Geometry: see drawing. Coordinates: mm, zero at the bounding-box minimum. Round coordinates to 2 decimals unless told otherwise and drop trailing zeros. Loops run counter-clockwise (first coordinate to the right, second up) from the corner with the lowest first, then second, coordinate; pieces in that order, holes last.
(1) Material intervals for probe 1 along X at (y, z) = (19, 93) (1 decimal); probe 2 along Z at (x, y) = (61, 16.5) (1 decimal); probe 3 along Z at (x, y) = (69, 3.5) (1 decimal), sorted ascending.
(2) Section B-B, the plane x = 38.5. Return the cut outline in (y, z), plus the area to 3 significant figures.
(3) Mould query, pull axis Z, two halves, no side actions, for the marked faces 1, 2 and 3. Classes: pulls with the +Z half, pulls with the -Z half, needs draft (parallel to the pull), parting line crosses it, or undercut.
(4) First-contact query: pin 1 Ø3 at (x, y) = (69.5, 21) entering from +Z; pin 2 Ø1 at (x, y) = (73, 17.5) entering from +Z; pin 3 Ø6 at (x, y) = (44.5, 28.5) entering from +Z. Flat tips, straight axial feed; report the tip coordinate or a pass-through.
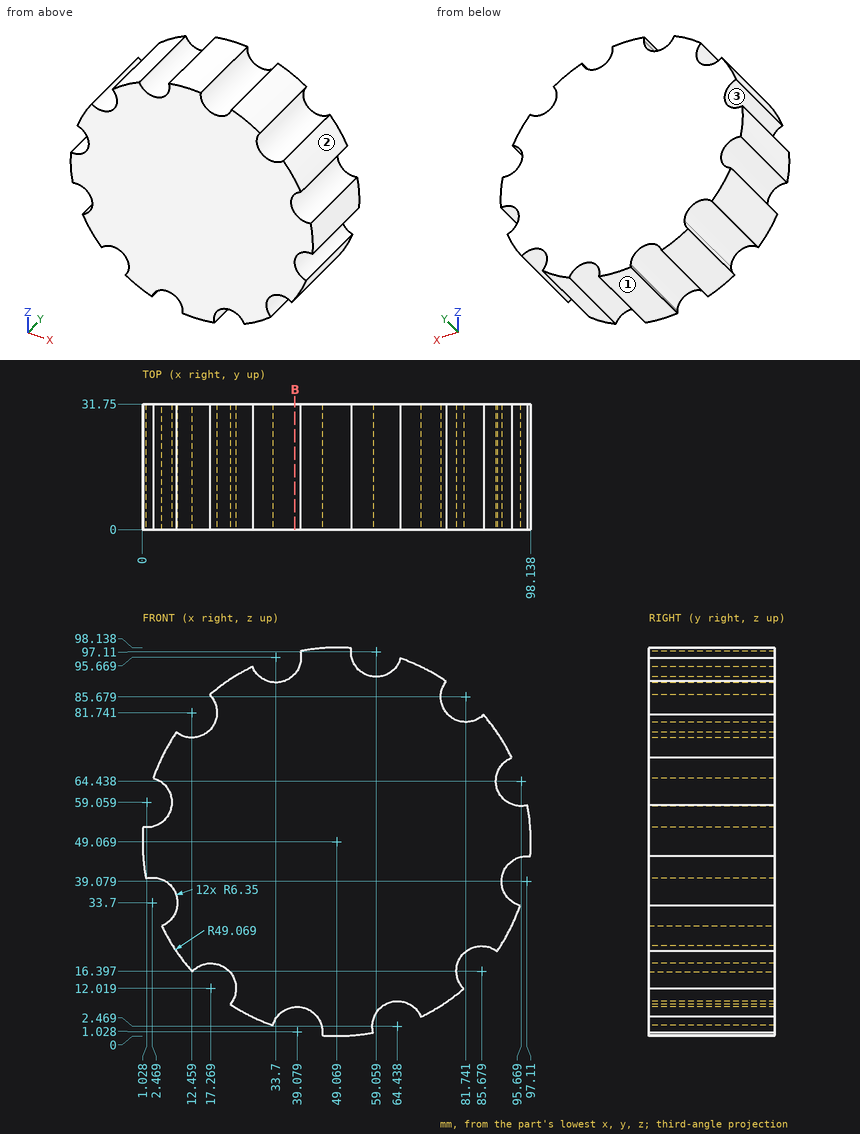
Output values:
1. probe 1: x = 27.2 to 27.9, 39.5 to 54.2, 63.9 to 70.9
1. probe 2: z = 7.8 to 91.1
1. probe 3: z = 6.9 to 93.9
2. outline: (0, 7.35) - (31.75, 7.35) - (31.75, 91.51) - (0, 91.51) - close
2. area: 2,670 mm2
3. face 1: pulls with the -Z half
3. face 2: pulls with the +Z half
3. face 3: undercut
4. pin 1: stops at z = 94.34
4. pin 2: stops at z = 92.18
4. pin 3: stops at z = 98.11
